Work out the finished part from the listing and answer in its coordinate system (mm). A direction names the side the tool comes from. Give positions to 0.01 mm unless a question says otherwise; leave off trailing zeros. Write each loop counter-clockwise with the first axis right and the second up, starting at its lowest first coordinate (ties: lowest second). Pieces come first, ordered by that corner, then holes. Notation, with made-up numbers: (-24.75, 62) -> (-7.75, 62) arc R25 cw to (-7.75, 74) -> close; hole circle Ø7 at (79.5, 75.25). An arc over 180 degrees is marked (long way). Use a Markdown table: item, result. Add a question column.
Q1. Consider line 1 (Z direction, x = 10.5, y = -1); line 2 (Y direction, x = 0.5, z = -76.5); line 3 (X direction, y = 5.5, z = -26.5). Determine where each line is inside the solid, lowest interval first.
Q2. Section B-B, the plane x = -9 is taken. Give the vertices of the cut face in (y, z).
Q3. Section C-C, the plane z = -28.5 is taken. Give the vertices of the cut face in (x, y).
Q4. Each of these flat-tipped pins is pushed along its axis until it touches: pin 1 Ø4 at (y, z) = (-2, -86.5) entering from +X; pin 2 Ø6 at (y, z) = (9.5, -92.5) entering from +X; pin 3 Ø3 at (y, z) = (-6, -64.5) entering from +X. Where does it stop, or does it pass through?
Q5. Section D-D, the plane y = 17.5 is taken. Give the vertices of the cut face in (x, z).
Q6. For faces 1 (the face through (-10.413, 0.115, -66.008)), 2 (the face through (0, 7.368, -66)), 3 (the face through (0, -7.368, -66)), 4 (the face through (10.413, -0.115, -66.008)), determine the directions among +Z, -Z, +X, -X, +Y, -Y from which every point of the face is accessible in a straight line to the end or side of a thin tool.
Q7. Section A-A, the plane y = 1 is taken. Give the vertices of the cut face in (x, z), plus the area to 3 significant figures.
from build123d import *

# Parameters (mm, degrees)
BOSS_EXTRUDE1_DEPTH = 114.3
BOSS_EXTRUDE2_DEPTH = 19.05


with BuildPart() as part:
    # Sketch1 → Boss-Extrude1 (new body)
    with BuildSketch(Plane.XY):
        with BuildLine():
            Line((-7.359452383, -7.368165079), (7.359452383, -7.368165079))
            ThreePointArc((7.359452383, -7.368165079), (10.414, 0), (7.359452383, 7.368165079))
            Line((7.359452383, 7.368165079), (-7.359452383, 7.368165079))
            ThreePointArc((-7.359452383, 7.368165079), (-10.414, 0), (-7.359452383, -7.368165079))
        make_face()
    extrude(amount=-BOSS_EXTRUDE1_DEPTH)

    # Sketch2 → Boss-Extrude2 (add)
    with BuildSketch(Plane.XY):
        with BuildLine():
            Line((2.171966529, 21.691427715), (23.229399553, -14.6453605))
            ThreePointArc((23.229399553, -14.6453605), (23.232480647, -17.187136052), (21.031750526, -18.458914093))
            Line((21.031750526, -18.458914093), (-21.582602225, -18.458914093))
            ThreePointArc((-21.582602225, -18.458914093), (-23.789789798, -17.175863979), (-23.767109444, -14.622947964))
            Line((-23.767109444, -14.622947964), (-2.210189717, 21.713840251))
            ThreePointArc((-2.210189717, 21.713840251), (-0.012691839, 22.957840901), (2.171966529, 21.691427715))
        make_face()
    extrude(amount=-BOSS_EXTRUDE2_DEPTH)


solid = part.part
Result set:
| question | item | result |
|---|---|---|
| 1 | line 1 | z = -19.05 to 0 |
| 1 | line 2 | y = -7.37 to 7.37 |
| 1 | line 3 | x = -8.84 to 8.84 |
| 2 | outline | (-18.46, -19.05) -> (-5.24, -19.05) -> (-5.24, -114.3) -> (5.24, -114.3) -> (5.24, -19.05) -> (10.27, -19.05) -> (10.27, 0) -> (-18.46, 0) -> close |
| 3 | outline | (-7.36, -7.37) -> (7.36, -7.37) arc R10.41 ccw to (7.36, 7.37) -> (-7.36, 7.37) arc R10.41 ccw to start |
| 4 | pin 1 | stops at x = 10.41 |
| 4 | pin 2 | stops at x = 8.14 |
| 4 | pin 3 | stops at x = 9.39 |
| 5 | outline | (-4.71, -19.05) -> (4.6, -19.05) -> (4.6, 0) -> (-4.71, 0) -> close |
| 6 | face 1 | -Z, -X |
| 6 | face 2 | -Z, +X, -X, +Y |
| 6 | face 3 | -Z, +X, -X, -Y |
| 6 | face 4 | -Z, +X |
| 7 | outline | (-14.5, -19.05) -> (-10.37, -19.05) -> (-10.37, -114.3) -> (10.37, -114.3) -> (10.37, -19.05) -> (14.16, -19.05) -> (14.16, 0) -> (-14.5, 0) -> close |
| 7 | area | 2,520 mm2 |
